Geometry check sheet. Reference: drawing and pictorial views, mm from the part's lowest x, y, z. A direction names the side the tool comes from. Give positions to 0.01 mm unless a question says otherwise; leave off trailing zeros. Write each loop counter-clockwise with the first axis right and the second up, starting at its lowest first coordinate (ties: lowest second). Pieces come first, ordered by that corner, then holes.
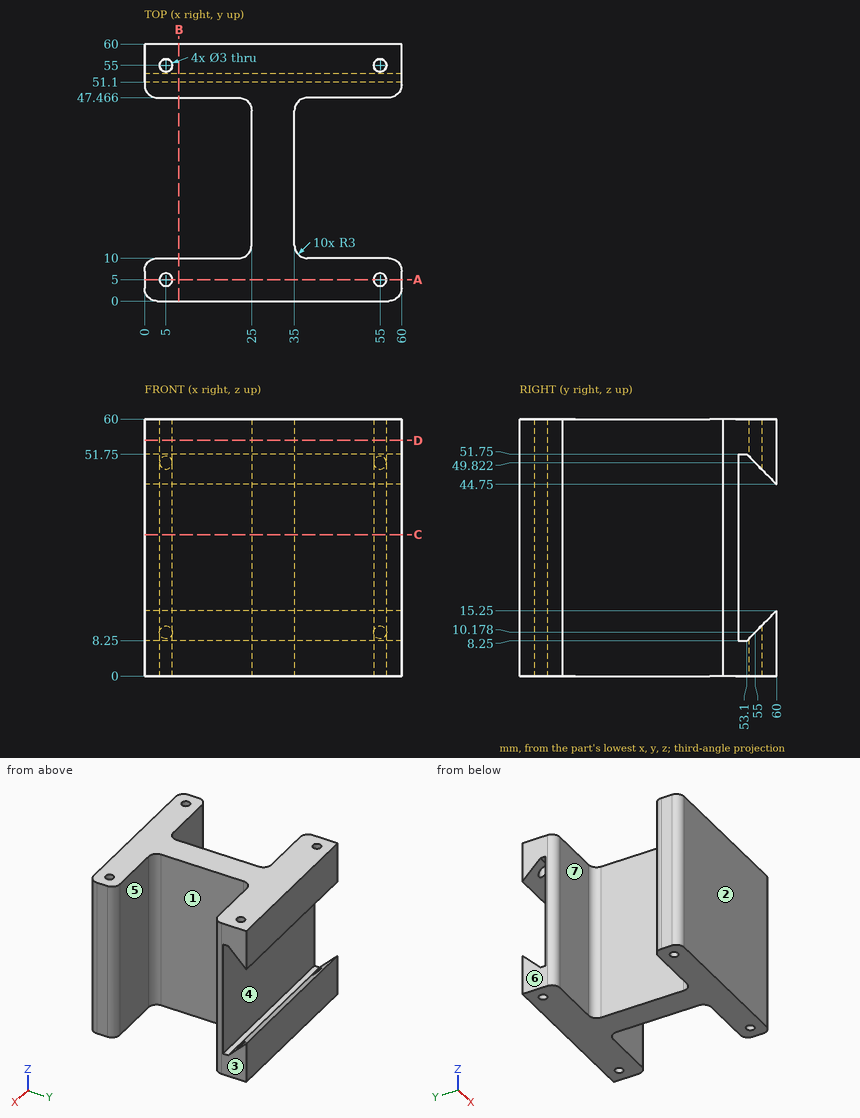
Item 1: Set-up check for the marked faces 4, 5, 6 and 7: record each of +Z, -Z, +X, -X, +Y, -Y from which the full face is reachable in a straight line by a thin tool's end or side.
Answer key:
face 4: +X, -X
face 5: +Z, -Z, +X
face 6: +Z, -Z, -X, +Y, -Y
face 7: +Z, -Z, -X
Item 2: Sectioned sample at B-B on x = 8. Record the cut outline in (y, z), then the cut area to 3 significant figures.
Answer key:
outline: (0, 0) - (10, 0) - (10, 60) - (0, 60) - close; (47.47, 0) - (60, 0) - (60, 15.25) - (53.1, 8.25) - (51.1, 8.25) - (51.1, 51.75) - (53.1, 51.75) - (60, 44.75) - (60, 60) - (47.47, 60) - close
area: 1,010 mm2
Item 3: Release check for a two-part mould opening along Y. For the marked faces 1, 2 and 3 record: released by +Y, released by -Y, zero draft, split by the parting line, or undercut.
Answer key:
face 1: undercut
face 2: released by -Y
face 3: zero draft
Item 4: Depth check by flat-ended pin: pin 1 (4 mm diameter, centred on x = 10, y = 44, fed in from -Z); pin 2 (12 mm diameter, centred on y = 33, z = 7.5, fed in from +X); pin 3 (9.5 mm diameter, centred on x = 11, z = 26.5, fed in from +Y). Enter the tip coordinate at first touch or a pass-through.
Answer key:
pin 1: passes through
pin 2: stops at x = 35
pin 3: stops at y = 51.1
Item 5: Sectioned sample at D-D on z = 55. Record the cut outline in (x, y), then the cut area to 3 significant figures.
Answer key:
outline: (0, 3) arc R3 ccw to (3, 0) - (57, 0) arc R3 ccw to (60, 3) - (60, 7) arc R3 ccw to (57, 10) - (38, 10) arc R3 cw to (35, 13) - (35, 44.47) arc R3 cw to (38, 47.47) - (57, 47.47) arc R3 ccw to (60, 50.47) - (60, 60) - (0, 60) - (0, 50.47) arc R3 ccw to (3, 47.47) - (22, 47.47) arc R3 cw to (25, 44.47) - (25, 13) arc R3 cw to (22, 10) - (3, 10) arc R3 ccw to (0, 7) - close; hole circle Ø3 at (5, 5); hole circle Ø3 at (5, 55); hole circle Ø3 at (55, 5); hole circle Ø3 at (55, 55)
area: 1,690 mm2
Item 6: Sectioned sample at A-A on y = 5. Record the cut outline in (x, z), then the cut area to 3 significant figures.
Answer key:
outline: (0, 0) - (3.5, 0) - (3.5, 60) - (0, 60) - close; (6.5, 0) - (53.5, 0) - (53.5, 60) - (6.5, 60) - close; (56.5, 0) - (60, 0) - (60, 60) - (56.5, 60) - close
area: 3,240 mm2
Item 7: Scan lines: line 1 along Y through (x, z) = (55, 57.5); line 2 along X through (y, z) = (55, 57.5); line 3 along Y through (x, z) = (5, 43). Record each from-to range of solid material in increasing order.
Answer key:
line 1: y = 0 to 3.5, 6.5 to 10, 47.47 to 53.5, 56.5 to 60
line 2: x = 0 to 3.5, 6.5 to 53.5, 56.5 to 60
line 3: y = 0 to 3.5, 6.5 to 10, 47.47 to 51.1
Item 8: Sectioned sample at C-C on z = 33. Record the cut outline in (x, y).
Answer key:
outline: (0, 3) arc R3 ccw to (3, 0) - (57, 0) arc R3 ccw to (60, 3) - (60, 7) arc R3 ccw to (57, 10) - (38, 10) arc R3 cw to (35, 13) - (35, 44.47) arc R3 cw to (38, 47.47) - (57, 47.47) arc R3 ccw to (60, 50.47) - (60, 51.1) - (0, 51.1) - (0, 50.47) arc R3 ccw to (3, 47.47) - (22, 47.47) arc R3 cw to (25, 44.47) - (25, 13) arc R3 cw to (22, 10) - (3, 10) arc R3 ccw to (0, 7) - close; hole circle Ø3 at (5, 5); hole circle Ø3 at (55, 5)
